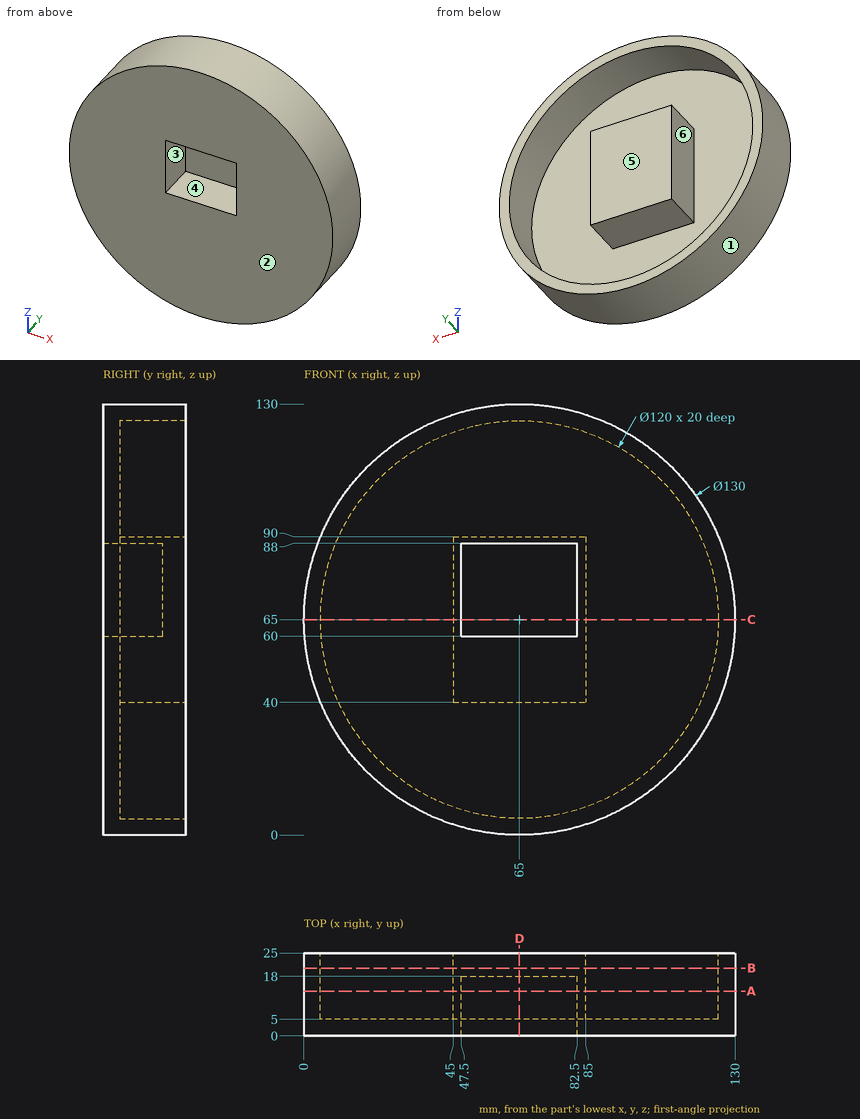
Here's the drawing with two shaded views (mm, measured from the low corner). I have some questions. A direction names the side the tool comes from. Give positions to 0.01 mm unless a question says otherwise; leave off trailing zeros. Order: outer loops, then holes, each group sorted by start corner. A loop starts at its lowest first (then second) coordinate and runs counter-clockwise, first axis right, second up. Notation, with made-up numbers: (-19.5, 47) -> (3.5, 47) arc R7 ccw to (3.5, 51) -> close; hole circle Ø2 at (56.5, -18.5). An arc over 180 degrees is marked (long way). One line per item, written item: value. Start each with the question number.
1. Will these pins go through, and if not, where does the flat tip stop? pin 1 Ø14 at (x, z) = (69.5, 69.5) entering from -Y; pin 2 Ø1 at (y, z) = (17.5, 80.5) entering from -X; pin 3 Ø12 at (y, z) = (10.5, 115) entering from +X.
2. Imagine slicing it at C-C, the plane z = 65. List the corners of the cut face in (x, y) for me.
3. Imagine slicing it at A-A, the plane y = 13.5. List the corners of the cut face in (x, z) for me, plus the area to 3 significant figures.
4. Imagine slicing it at D-D, the plane x = 65. List the corners of the cut face in (y, z) for me, plus the area to 3 significant figures.
5. I need wall thicknesses on probe 1 along X at (y, z) = (13, 65); probe 2 along X at (y, z) = (20.25, 65); probe 3 along X at (y, z) = (20.25, 59.5). Which ranges of each line are inside material? Lowest first, please. Write a range as from..to.
6. For the marked faces 4, 5 and 6, which set-ups out of +Z, -Z, +X, -X, +Y, -Y let a thin tool reach every point of the face, with its end or its side?
7. Imagine slicing it at B-B, the plane y = 20.5. List the corners of the cut face in (x, z) for me.
8. We'd pull the mould along X, two halves only. Please class the marked faces 1, 2 and 3: released by +X, released by -X, zero draft, split by the parting line, or undercut.
Values follow:
1. pin 1: stops at y = 18
1. pin 2: stops at x = 1.75
1. pin 3: stops at x = 112.84
2. outline: (0, 0) -> (47.5, 0) -> (47.5, 18) -> (82.5, 18) -> (82.5, 0) -> (130, 0) -> (130, 25) -> (125, 25) -> (125, 5) -> (85, 5) -> (85, 25) -> (45, 25) -> (45, 5) -> (5, 5) -> (5, 25) -> (0, 25) -> close
3. outline: circle Ø130 at (65, 65); (45, 40) -> (85, 40) -> (85, 90) -> (45, 90) -> close; hole circle Ø120 at (65, 65); hole (47.5, 60) -> (82.5, 60) -> (82.5, 88) -> (47.5, 88) -> close
3. area: 2,980 mm2
4. outline: (0, 0) -> (25, 0) -> (25, 5) -> (5, 5) -> (5, 40) -> (25, 40) -> (25, 90) -> (5, 90) -> (5, 125) -> (25, 125) -> (25, 130) -> (0, 130) -> (0, 88) -> (18, 88) -> (18, 60) -> (0, 60) -> close
4. area: 1,350 mm2
5. probe 1: x = 0..5, 45..47.5, 82.5..85, 125..130
5. probe 2: x = 0..5, 45..85, 125..130
5. probe 3: x = 0.23..5.25, 45..85, 124.75..129.77
6. face 4: -Y
6. face 5: +Z, -Z, +X, -X, +Y
6. face 6: +Y
7. outline: circle Ø130 at (65, 65); (45, 40) -> (85, 40) -> (85, 90) -> (45, 90) -> close; hole circle Ø120 at (65, 65)
8. face 1: split by the parting line
8. face 2: zero draft
8. face 3: undercut
